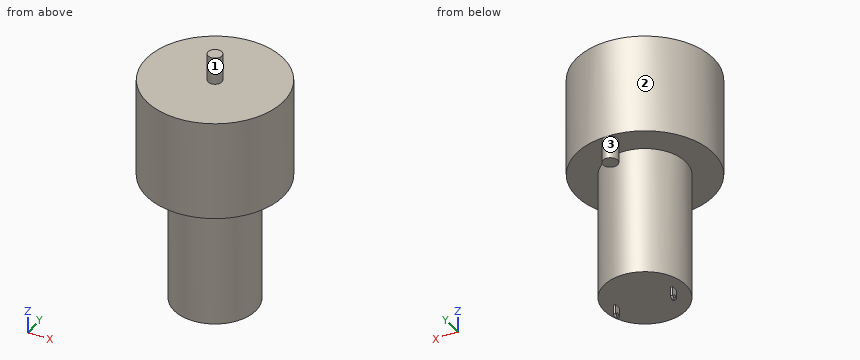
from build123d import *

# Parameters (mm, degrees)
SKETCH_5_R      = 3.25
EXTRUDE_1_DEPTH = 10
EXTRUDE_START   = 12
SKETCH_7_R      = 0.677279549
EXTRUDE_2_DEPTH = 1


with BuildPart() as part:
    # 草图4 → 旋转1 (revolve)
    with BuildSketch(Plane(origin=(0, 0, 0), x_dir=(0, 0, -1), z_dir=(1, 0, 0)), mode=Mode.PRIVATE) as revolve_1_sk:
        Polygon((0, 0), (112, 0), (112, 17.9), (55.5, 17.9), (55.5, 30), (12, 30), (12, 3), (0, 3), align=None)
    revolve(revolve_1_sk.sketch.rotate(Axis((0, 0, 0), (0, 0, -1)), 90), axis=Axis((0, 0, 0), (0, 0, -1)))

    # 草图5 → 凸台-拉伸1 (add)
    with BuildSketch(Plane(origin=(0, 0, -55.5), x_dir=(-1, 0, 0), z_dir=(0, 0, -1))):
        with Locations(Location((0, 26.75, 0), (0, 0, 90))):
            Circle(SKETCH_5_R)
    extrude(amount=EXTRUDE_1_DEPTH)

    # 草图7 → 凸台-拉伸2 (add)
    with BuildSketch(Plane(origin=(0, 0, 0), x_dir=(0, 0, -1), z_dir=(1, 0, 0)).offset(EXTRUDE_START)):
        Polygon((112, 0), (112, 1.5), (116, 1.5), (117, 0.5), (117, -0.5), (116, -1.5), (112, -1.5), align=None)
        with Locations((115.558241223, 0)):
            Circle(SKETCH_7_R, mode=Mode.SUBTRACT)
    extrude_2 = extrude(amount=EXTRUDE_2_DEPTH)

    # 镜向1: 凸台-拉伸2 across plane
    add(extrude_2.mirror(Plane(origin=(0, 0, 0), x_dir=(0, 0, 1), z_dir=(1, 0, 0))))


solid = part.part
The listing builds one solid part. Answer for the finished solid, in the listing's coordinates (mm). Face numbers are marked on the shaded views. A direction names the side the tool comes from. Coordinates: 2 decimals unless noted, no trailing zeros. Write each loop counter-clockwise with the first axis right and the second up, starting at its lowest first coordinate (ties: lowest second). Pieces come first, ordered by that corner, then holes. Notation, with made-up numbers: M 65,56.5 L 104,56.5 A21 ccw 104,78.5 Z; hole C 62,55 d3. An arc over 180 degrees is marked long. Use one line per item in the form item = value.
Item 1: Find the intervals of material crossed by probe 1 along Z at (x, y) = (26, -1.5); probe 2 along Z at (x, y) = (-12, -2.5); probe 3 along X at (y, z) = (-0.5, -77.5), in increasing order.
Model answer:
probe_1 = -55.5 to -12
probe_2 = -112 to -12
probe_3 = -17.89 to 17.89
Item 2: For the marked faces 1, 2 and 3, determine the directions among +Z, -Z, +X, -X, +Y, -Y from which every point of the face is accessible in a straight line to the end or side of a thin tool.
Model answer:
face_1 = +Z
face_2 = +Z, -Z
face_3 = -Z
Item 3: Find section D-D, the plane z = -42. Give the vertices of the cut face in (x, y), plus the area to 3 significant figures.
Model answer:
outline = C 0,0 d60
area = 2,830 mm2
Item 4: Given P1, Ø2.5, axis at y = 0.5, z = -114, coming from the -X side; P2, Ø1.1, axis at x = -12.5, z = -113.5, coming from the +Y side; P3, Ø12, axis at x = -18.5, y = 15.5, coming from the +Z side; P4, Ø0.8, axis at y = 0, z = -115.56, coming from the -X side, each flat-ended and moving along its own axis, determine where each tip first touches the part or whether it passes through.
Model answer:
P1 = -13
P2 = 1.5
P3 = -12
P4 = through
Item 5: Find section A-A, the plane z = -58. Give the vertices of the cut face in (x, y), plus the area to 3 significant figures.
Model answer:
outline = C 0,0 d35.8; C 0,26.75 d6.5
area = 1,040 mm2
Item 6: Find section B-B, the plane x = -10.5. Give the vertices of the cut face in (y, z).
Model answer:
outline = M -28.1,-55.5 L -14.5,-55.5 L -14.5,-112 L 14.5,-112 L 14.5,-55.5 L 28.1,-55.5 L 28.1,-12 L -28.1,-12 Z
Item 7: Find section C-C, the plane y = -6.5. Give the vertices of the cut face in (x, z), plus the area to 3 significant figures.
Model answer:
outline = M -29.29,-55.5 L -16.68,-55.5 L -16.68,-112 L 16.68,-112 L 16.68,-55.5 L 29.29,-55.5 L 29.29,-12 L -29.29,-12 Z
area = 4,430 mm2
